Here's how the part is built. I have some questions about the finished solid (model axes, mm). A direction names the side the tool comes from. Give positions to 0.01 mm unless a question says otherwise; leave off trailing zeros. Order: outer loops, then holes, each group sorted by start corner. A loop starts at its lowest first (then second) coordinate and runs counter-clockwise, first axis right, second up. Notation, with made-up numbers: (-35.75, 2) - (-0.75, 2) arc R22 cw to (-0.75, 27) - close; hole circle Ø8 at (-25, 59.5). An arc over 180 degrees is marked (long way). One line per question, with ' | ' between items.
from build123d import *

# Parameters (mm, degrees)
F4_W     = 3
F4_H     = 9
F5_DEPTH = 25


with BuildPart() as f3:
    # F0 (on Top) → F3 section 0
    with BuildSketch(Plane.XY):
        Polygon((-35.883552, 29.228954), (-20.883552, 29.228954), (-20.883552, -138.771046), (12.616448, -138.771046), (12.616448, -98.771046), (4.616448, -98.771046), (4.616448, -132.771046), (-15.883552, -132.771046), (-15.883552, 42.228954), (-35.883552, 42.228954), align=None)
    # F2 (on offset) → F3 section 1
    with BuildSketch(Plane.XY.offset(19)):
        Polygon((-35.883552, 29.228954), (-25.883552, 29.228954), (-25.883552, -138.771046), (7.616448, -138.771046), (7.616448, -98.771046), (-0.383552, -98.771046), (-0.383552, -132.771046), (-20.883552, -132.771046), (-20.883552, 42.228954), (-35.883552, 42.228954), align=None)
    loft()

    # F4 (on face) → F5 (cut)
    with BuildSketch(Plane.XY.offset(19)):
        with Locations((-27.383552, 33.728954)):
            Rectangle(F4_W, F4_H)
    extrude(amount=-F5_DEPTH, mode=Mode.SUBTRACT)


solid = f3.part
1) I want a section at A-A (y = -104.5). List the corners of the cut face in (x, z) for me.
Model answer:
outline: (-25.88, 19) - (-20.88, 0) - (-15.88, 0) - (-20.88, 19) - close; (-0.38, 19) - (4.62, 0) - (12.62, 0) - (7.62, 19) - close
2) Thinking about a two-plate mould opening in X: for faces 1 (the face through (-23.419, -53.595, 9.633)), 2 (the face through (-16.2, -63.6, 0)), 3 (the face through (-27, 38.229, 10)), which applies, +X half, -X half, draft (parallel to the pull), parting line (faces both ways), or undercut?
Model answer:
face 1: -X half | face 2: draft | face 3: undercut
3) On a 3-axis mill with a long thin cutter (end or side, diameter ignored), from which of +Z, -Z, +X, -X, +Y, -Y can I reach the whole of each face in a straight line? I mean faces 4 (the face through (-35.884, 36, 10)), 5 (the face through (-18.419, -46.496, 9.633)), 6 (the face through (-25.884, 34, 10)), 7 (the face through (2.081, -115.533, 9.633)). Say none if no direction works.
Model answer:
face 4: +Z, -Z, -X, +Y, -Y | face 5: +Z, +Y | face 6: +Z, -Z, -Y | face 7: -Z, +Y
4) Please list where these lines run through material, in increasing order: L1, parallel to Y at x = -27, z = 5.5; L2, parallel to X at y = -108, z = 4.25; L3, parallel to Y at x = -12.5, z = 6.5.
Model answer:
L1: y = 38.23 to 42.23 | L2: x = -22 to -17, 3.5 to 11.5 | L3: y = -138.77 to -132.77
5) I want a section at B-B (y = 21). List the corners of the cut face in (x, z) for me, plus the area to 3 significant figures.
Model answer:
outline: (-25.88, 19) - (-20.88, 0) - (-15.88, 0) - (-20.88, 19) - close | area: 95.0 mm2
6) I'm going to push flat-ended pins straight in: P1, Ø4.5, axis at y = 32, z = 10.5, coming from the +X side; P2, Ø8, axis at y = 10.5, z = 15, coming from the +X side; P3, Ø3.5, axis at x = -27.5, z = 6.5, coming from the -Y side. Where does each tip first touch, or does it pass through?
Model answer:
P1: stops at x = -18.05 | P2: stops at x = -18.78 | P3: stops at y = 29.23
